```python
from build123d import *

# Parameters (mm, degrees)
SKETCH1_R           = 4
SKETCH1_R_2         = 3
BOSS_EXTRUDE1_DEPTH = 2
FILLET1_R           = 1


with BuildPart() as part:
    # Sketch1 → Boss-Extrude1 (new body)
    # profile 1 of 3: a face of its own
    with BuildSketch(Plane(origin=(0, 0, 0), x_dir=(1, 0, 0), z_dir=(0, 1, 0))):
        with Locations((0, 11.25)):
            Circle(SKETCH1_R)
        with Locations(Location((0, 11.25, 0), (0, 0, 270))):
            Circle(SKETCH1_R_2, mode=Mode.SUBTRACT)
    # profile 2 of 3: a face of its own
    with BuildSketch(Plane(origin=(0, 0, 0), x_dir=(1, 0, 0), z_dir=(0, 1, 0))):
        with BuildLine():
            Line((-1, 7.377016654), (-1, -7.377016654))
            ThreePointArc((-1, -7.377016654), (0, -7.25), (1, -7.377016654))
            Line((1, -7.377016654), (1, 7.377016654))
            ThreePointArc((1, 7.377016654), (0, 7.25), (-1, 7.377016654))
        make_face()
    # profile 3 of 3: a face of its own
    with BuildSketch(Plane(origin=(0, 0, 0), x_dir=(1, 0, 0), z_dir=(0, 1, 0))):
        with Locations((0, -11.25)):
            Circle(SKETCH1_R)
        with Locations(Location((0, -11.25, 0), (0, 0, 270))):
            Circle(SKETCH1_R_2, mode=Mode.SUBTRACT)
    extrude(amount=BOSS_EXTRUDE1_DEPTH)

    # Fillet1
    fillet1_edges = [part.edges().sort_by_distance(p)[0] for p in [
        (1, 1, -7.377016654),
        (1, 1, 7.377016654),
        (-1, 1, 7.377016654),
        (-1, 1, -7.377016654),
    ]]
    fillet(fillet1_edges, radius=FILLET1_R)


solid = part.part
```
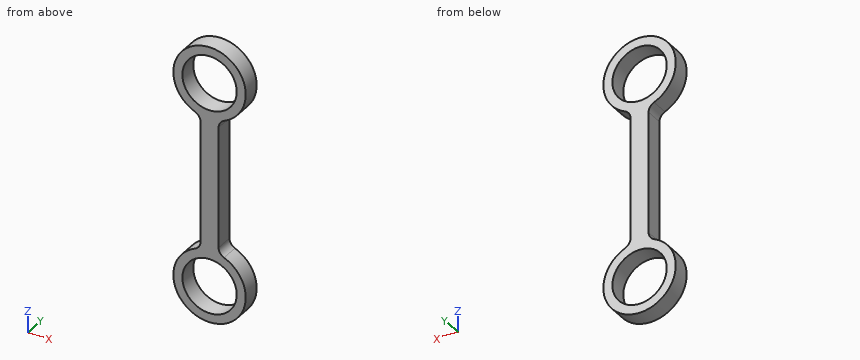
Input: part model. Units: mm. Frame: model coordinates. Give positions to 0.01 mm unless a question says otherwise; leave off trailing zeros. Order: outer loops, then holes, each group sorted by start corner. A loop starts at its lowest first (then second) coordinate and runs counter-clockwise, first axis right, second up.
1. Section A-A on z = 11.25. Return the cut outline in (x, y), and give its area (3 significant figures).
Derived:
outline: (-4, 0) - (-3, 0) - (-3, 2) - (-4, 2) - close; (3, 0) - (4, 0) - (4, 2) - (3, 2) - close
area: 4.00 mm2
2. Section B-B on x = -0.5. Return the cut outline in (y, z), and give its area (3 significant figures).
Derived:
outline: (0, -15.22) - (2, -15.22) - (2, -14.21) - (0, -14.21) - close; (0, -8.29) - (2, -8.29) - (2, 8.29) - (0, 8.29) - close; (0, 14.21) - (2, 14.21) - (2, 15.22) - (0, 15.22) - close
area: 37.2 mm2
3. Pin query (flat end, axial travel): pin 1 (1 mm diameter, centred on y = 1, z = -2.5, fed in from -X); pin 2 (1 mm diameter, centred on y = 0.5, z = -0.5, fed in from +X). Return the tip coordinate at first contact, or that it passes through.
Derived:
pin 1: stops at x = -1
pin 2: stops at x = 1
4. Section C-C on y = 1.3. Return the cut outline in (x, z).
Derived:
outline: (-1.6, -7.58) arc R4 ccw (long way) to (1.6, -7.58) arc R1 cw to (1, -6.67) - (1, 6.67) arc R1 cw to (1.6, 7.58) arc R4 ccw (long way) to (-1.6, 7.58) arc R1 cw to (-1, 6.67) - (-1, -6.67) arc R1 cw to start; hole circle Ø6 at (0, -11.25); hole circle Ø6 at (0, 11.25)
5. Section D-D on z = -9. Return the cut outline in (x, y).
Derived:
outline: (-3.31, 0) - (-1.98, 0) - (-1.98, 2) - (-3.31, 2) - close; (1.98, 0) - (3.31, 0) - (3.31, 2) - (1.98, 2) - close
6. Material intervals for L1, parallel to X at y = 1.2, z = -11.25; L2, parallel to Z at x = -0.75, y = 0.3; L3, parallel to Z at x = 1.75, y = 1.6, sorted ascending.
Derived:
L1: x = -4 to -3, 3 to 4
L2: z = -15.18 to -14.15, -8.35 to 8.35, 14.15 to 15.18
L3: z = -14.85 to -13.69, -8.81 to -7.65, 7.65 to 8.81, 13.69 to 14.85
